Geometry: final body of the model. Coordinates: model frame, mm. A direction names the side the tool comes from. Coordinates: 2 decimals unless noted, no trailing zeros. Order: outer loops, then holes, each group sorted by start corner. A loop starts at its lowest first (then second) coordinate and runs counter-clockwise, first axis right, second up. Notation, with made-up numbers: (69.5, 7.5) -> (104.5, 7.5) arc R31 ccw to (104.5, 37.5) -> close; hole circle Ø11 at (62, 89.25). An arc over 180 degrees is marked (long way). Answer in a Markdown table with one row per item. Add a question column.
1) Section query C-C on y = 44. Return the cut outline in (x, z).
2) Section query D-D on x = 212. Return the cut outline in (y, z).
3) Set-up query: faces 1 (the face through (152, 101.6, -50)), 2 (the face through (152, 121, 25.4)), 3 (the face through (151, 50.8, 51)), 4 (the face through (229.7, 75.1, 1.1)), 5 (the face through (151, 50.8, -50)). Return all of +Z, -Z, +X, -X, +Y, -Y with unobstructed straight access to the full face (end or side cutting, diameter ignored); none if empty.
4) Section query A-A on x = 80. Return the cut outline in (y, z), then the cut area to 3 significant figures.
5) Contact query for flat-ended pins moving along their axis: P1, Ø15, axis at x = 106, z = -59, coming from the -Y side; P2, Ø4, axis at y = 28.5, z = 13, coming from the -X side; P3, Ø15, axis at x = 152.5, z = -45, coming from the +Y side; P4, Ø2, axis at x = 259, z = 28, coming from the -Y side. Output: stop coordinate, or through.
6) Ray query, line 1 (Y direction, x = 110, z = -28); line 2 (Z direction, x = 32.5, y = 25.5); line 3 (Y direction, x = 218, z = -21.5). Return the intervals inside material, ascending. Write a range as from..to.
```python
from build123d import *

# Parameters (mm, degrees)
SKETCH1_W           = 50.8
SKETCH1_H           = 152.4
SKETCH1_W_2         = 152.4
SKETCH1_H_2         = 50.8
EXTRUDE_THIN1_DEPTH = 304.8
CHAMFER1_SIZE       = 152.4


with BuildPart() as part:
    # Sketch1 → Extrude-Thin1 (new body)
    with BuildSketch(Plane(origin=(0, 0, 0), x_dir=(0, 0, -1), z_dir=(1, 0, 0))):
        with Locations((0, 76.2)):
            Rectangle(SKETCH1_W, SKETCH1_H)
        with Locations((0, 76.2)):
            Rectangle(SKETCH1_W_2, SKETCH1_H_2)
    extrude(amount=EXTRUDE_THIN1_DEPTH)

    # Chamfer1
    chamfer1_edges = [part.edges().sort_by_distance(p)[0] for p in [
        (304.8, 152.4, 0),
        (0, 152.4, 0),
    ]]
    chamfer(chamfer1_edges, length=CHAMFER1_SIZE - 0.0001)  # a hair under: the kernel refuses the full size


solid = part.part
```
Result:
| question | item | result |
|---|---|---|
| 1 | outline | (44, -25.4) -> (260.8, -25.4) -> (260.8, 25.4) -> (44, 25.4) -> close |
| 2 | outline | (0, -25.4) -> (50.8, -25.4) -> (50.8, -76.2) -> (92.8, -76.2) -> (92.8, 76.2) -> (50.8, 76.2) -> (50.8, 25.4) -> (0, 25.4) -> close |
| 3 | face 1 | -Z, +X, -X, +Y |
| 3 | face 2 | +Z, +X, -X, +Y |
| 3 | face 3 | +Z, +X, -X, -Y |
| 3 | face 4 | +Z, -Z, +X, +Y |
| 3 | face 5 | -Z, +X, -X, -Y |
| 4 | outline | (0, -25.4) -> (50.8, -25.4) -> (50.8, -76.2) -> (80, -76.2) -> (80, 76.2) -> (50.8, 76.2) -> (50.8, 25.4) -> (0, 25.4) -> close |
| 4 | area | 7,030 mm2 |
| 5 | P1 | y = 50.8 |
| 5 | P2 | x = 26.5 |
| 5 | P3 | y = 101.6 |
| 5 | P4 | through |
| 6 | line 1 | 50.8..101.6 |
| 6 | line 2 | -25.4..25.4 |
| 6 | line 3 | 0..86.8 |
